Autodesk Inventor part; units mm, degrees
ref_plane "YZ Plane" through (0, 0, 0) normal (1, 0, 0) x (0, 1, 0)
ref_plane "XZ Plane" through (0, 0, 0) normal (0, 1, 0) x (-1, 0, 0)
ref_plane "XY Plane" through (0, 0, 0) normal (0, 0, 1) x (1, 0, 0)
sketch "Sketch1" plane through (0, 0, 0) normal (0, 1, 0) x (-1, 0, 0)
  point P0 (0, 0)
sketch "Sketch2" plane through (0, 0, 0) normal (0, 1, 0) x (-1, 0, 0)
  circle A0 centre (0, 0) radius 4.7625
  circle A1 centre (20.32, 0) radius 40
  line L0 (20.32, -34.925) -> (20.32, 34.925) construction
  line L1 (29.845, -25.4) -> (29.845, 25.4) construction
  line L2 (10.795, 25.4) -> (10.795, -25.4) construction
  arc A2 (10.795, -25.4) -> (29.845, -25.4) centre (20.32, -25.4) ccw construction
  arc A3 (29.845, 25.4) -> (10.795, 25.4) centre (20.32, 25.4) ccw construction
  line L3 (-19.68, 0) -> (60.32, 0) construction
  circle A4 centre (0, 0) radius 20.32 construction
  circle A5 centre (40.64, 0) radius 20.32 construction
  circle A6 centre (20.32, 0) radius 40.64 construction
  line L4 (20.32, 0) -> (48.6043, -28.2843) construction
  line L5 (20.32, 0) -> (60.32, 0) construction
  circle A7 centre (45.1244, -24.8044) radius 2.3812
  circle A8 centre (45.1244, -24.8044) radius 4.9212 construction
  circle A9 centre (45.1244, 24.8044) radius 2.3812
  circle A10 centre (-4.4844, 24.8044) radius 2.3812
  circle A11 centre (-4.4844, -24.8044) radius 2.3812
  line L6 (43.9547, -3.3147) -> (37.3253, -3.3147)
  line L7 (37.3253, -3.3147) -> (37.3253, 3.3147)
  line L8 (37.3253, 3.3147) -> (43.9547, 3.3147)
  line L9 (43.9547, 3.3147) -> (43.9547, -3.3147)
  line L10 (43.9547, -3.3147) -> (37.3253, 3.3147) construction
  line L11 (37.3253, -3.3147) -> (43.9547, 3.3147) construction
  circle A12 centre (40.64, 0) radius 5.0254
  dimension "d5" = 40.64
  dimension "d0" = 9.525
  dimension "d1" = 80
  dimension "d2" = 19.05
  dimension "d3" = 69.85
  dimension "d6" = 81.28
  dimension "d7" = 45
  dimension "d8" = 4.7625
  dimension "d9" = 2.54
  dimension "d12" = 360
  dimension "d16" = 6.6294
  dimension "d18" = 10.0508
extrude "Extrusion1" add sketch "Sketch2" along normal blind 6.35 contours A1 | A12
sketch "Sketch3" plane through (-20.32, 6.35, 0) normal (0, 1, 0) x (1, 0, 0)
  circle A0 centre (-20.32, 0) radius 5.0254
  point P0 (20.32, 0)
  dimension "d19" = 10.0508
extrude "Extrusion2" cut sketch "Sketch3" against normal blind 2
properties part number "carriage"
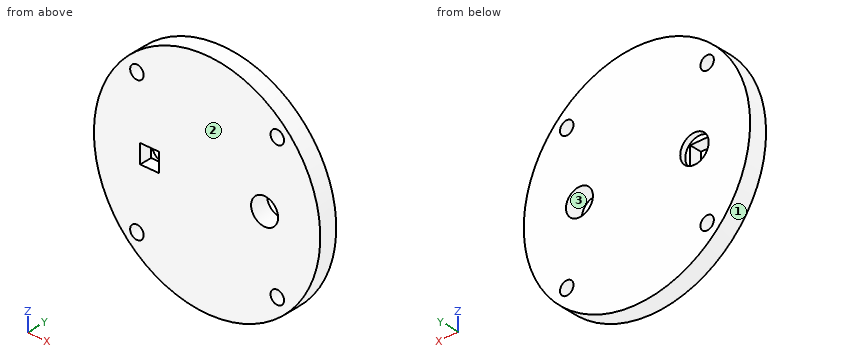
The listing builds one solid part. Answer for the finished solid, in the listing's coordinates (mm). Face numbers are marked on the shaded views. Round coordinates to 2 decimals unless told otherwise and drop trailing zeros. Order: outer loops, then holes, each group sorted by start corner. A loop starts at its lowest first (then second) coordinate and runs counter-clockwise, first axis right, second up. Notation, with made-up numbers: (-25, -26) -> (-10, -26) arc R15 cw to (-10, -12) -> close; hole circle Ø10 at (-16.5, 54.5). An arc over 180 degrees is marked (long way). One line per item, written item: value.
Item 1: Find section A-A, the plane z = 0. Give the vertices of the cut face in (x, y), then the cut area to 3 significant figures.
Taken from the geometry:
outline: (-60.32, 0) -> (-43.95, 0) -> (-43.95, 4.35) -> (-45.67, 4.35) -> (-45.67, 6.35) -> (-60.32, 6.35) -> close; (-37.33, 0) -> (-4.76, 0) -> (-4.76, 6.35) -> (-35.61, 6.35) -> (-35.61, 4.35) -> (-37.33, 4.35) -> close; (4.76, 0) -> (19.68, 0) -> (19.68, 6.35) -> (4.76, 6.35) -> close
area: 399 mm2
Item 2: Given P1, Ø9, axis at x = -40.64, z = 0, coming from the +Y side; P2, Ø3, axis at x = 4.48, z = -24.8, coming from the +Y side; P3, Ø3.5, axis at x = -40.5, y = 2.5, coming from the -Z side; P4, Ø1.3, axis at x = -42, y = 1.5, coming from the +Z side, each flat-ended and moving along its own axis, determine where each tip first touches the part or whether it passes through.
Taken from the geometry:
P1: stops at y = 4.35
P2: passes through
P3: stops at z = -35.5
P4: stops at z = 34.03
Item 3: Find section D-D, the plane z = 14. Give the vertices of the cut face in (x, y).
Taken from the geometry:
outline: (-57.79, 0) -> (17.15, 0) -> (17.15, 6.35) -> (-57.79, 6.35) -> close
Item 4: Find section B-B, the plane x = -40.64. Give the vertices of the cut face in (y, z).
Taken from the geometry:
outline: (0, -34.45) -> (6.35, -34.45) -> (6.35, -5.03) -> (4.35, -5.03) -> (4.35, -3.31) -> (0, -3.31) -> close; (0, 3.31) -> (4.35, 3.31) -> (4.35, 5.03) -> (6.35, 5.03) -> (6.35, 34.45) -> (0, 34.45) -> close
Item 5: Find section C-C, the plane y = 2. Give the vertices of the cut face in (x, z) (1 decimal).
Taken from the geometry:
outline: circle Ø80 at (-20.3, 0); hole circle Ø4.8 at (-45.1, -24.8); hole circle Ø4.8 at (-45.1, 24.8); hole (-44, -3.3) -> (-37.3, -3.3) -> (-37.3, 3.3) -> (-44, 3.3) -> close; hole circle Ø9.5 at (0, 0); hole circle Ø4.8 at (4.5, -24.8); hole circle Ø4.8 at (4.5, 24.8)
Item 6: For a pull along Z with two mould halves and no side action, classify the marked faces 1, 2 and 3 as released by +Z, released by -Z, zero draft, split by the parting line, or undercut.
Taken from the geometry:
face 1: split by the parting line
face 2: zero draft
face 3: undercut
Item 7: Straight lines are drawn through the part: L1, parallel to Z at x = -44.5, y = 2.5; L2, parallel to X at y = 6.25, z = 1; L3, parallel to Z at x = 6.5, y = 4. For each, find the intervals that lie inside material, in ascending order.
Taken from the geometry:
L1: z = -31.86 to -27.1, -22.51 to 22.51, 27.1 to 31.86
L2: x = -60.31 to -45.56, -35.72 to -4.66, 4.66 to 19.67
L3: z = -29.68 to -26.07, -23.54 to 23.54, 26.07 to 29.68
